```python
from build123d import *

# Parameters (mm, degrees)
BOSS_EXTRUDE1_DEPTH = 50.8
DRAFT1_ANGLE        = 2.86
CUT_EXTRUDE1_DEPTH  = 10.16
SKETCH3_W           = 20.078449586
SKETCH3_H           = 5.08
BOSS_EXTRUDE2_DEPTH = 12.7
CUT_EXTRUDE2_START  = -28.101341283
SKETCH4_R           = 1.905
SKETCH4_W           = 5.08
SKETCH4_H           = 14.732
CUT_EXTRUDE2_DEPTH  = 34.466005054
SKETCH5_W           = 15.24
SKETCH5_H           = 14.732
CUT_EXTRUDE3_DEPTH  = 6.35


with BuildPart() as part:
    # Sketch1 → Boss-Extrude1 (new body)
    with BuildSketch(Plane(origin=(0, 0, 0), x_dir=(1, 0, 0), z_dir=(0, 1, 0))):
        Polygon((-20.199224793, 2.212174897), (0, 0), (20.199224793, 2.212174897), (20.199224793, 22.532174897), (-20.199224793, 22.532174897), align=None)
    extrude(amount=-BOSS_EXTRUDE1_DEPTH)

    # Draft1
    draft1_faces = [part.faces().sort_by_distance(p)[0] for p in [
        (10.099612396, -25.4, -1.106087448),
        (-10.099612396, -25.4, -1.106087448),
    ]]
    draft(draft1_faces, Plane(origin=(0, -50.8, 0), x_dir=(0, 0, -1), z_dir=(0, -1, 0)), DRAFT1_ANGLE)

    # Sketch2 → Cut-Extrude1 (cut)
    with BuildSketch(Plane.ZY.offset(20.199224793)):
        Polygon((-22.532174897, -30.48), (-2.212174897, -50.8), (-22.532174897, -50.8), align=None)
    cut_extrude1 = extrude(amount=-CUT_EXTRUDE1_DEPTH, mode=Mode.SUBTRACT)

    # Mirror1: Cut-Extrude1 across plane
    add(cut_extrude1.mirror(Plane.ZY), mode=Mode.SUBTRACT)

    # Sketch3 → Boss-Extrude2 (add)
    with BuildSketch(Plane.XZ.offset(50.8)):
        with Locations((0, -19.992174897)):
            Rectangle(SKETCH3_W, SKETCH3_H)
    extrude(amount=BOSS_EXTRUDE2_DEPTH)

    # Sketch4 → Cut-Extrude2 (cut)
    with BuildSketch(Plane(origin=(-0.275601276, -0.126470659, 2.516497283), x_dir=(0.99407118, -0.005457579, 0.108594221), z_dir=(-0.108731274, -0.04989569, 0.992818176)).offset(CUT_EXTRUDE2_START)):
        with Locations((-9.882603301, -15.834429405)):
            Circle(SKETCH4_R)
        with Locations((-9.882603301, -34.884429405)):
            Circle(SKETCH4_R)
        with Locations((-4.802603301, -25.359429405)):
            Rectangle(SKETCH4_W, SKETCH4_H)
    cut_extrude2 = extrude(amount=CUT_EXTRUDE2_DEPTH, mode=Mode.SUBTRACT)

    # Sketch5 → Cut-Extrude3 (cut)
    with BuildSketch(Plane(origin=(-0.275601276, -0.126470659, 2.516497283), x_dir=(0.99407118, -0.005457579, 0.108594221), z_dir=(-0.108731274, -0.04989569, 0.992818176))):
        with Locations((-9.882603301, -25.359429405)):
            Rectangle(SKETCH5_W, SKETCH5_H)
    cut_extrude3 = extrude(amount=-CUT_EXTRUDE3_DEPTH, mode=Mode.SUBTRACT)

    # Mirror2: Cut-Extrude2, Cut-Extrude3 across plane
    add(cut_extrude2.mirror(Plane.ZY), mode=Mode.SUBTRACT)
    add(cut_extrude3.mirror(Plane.ZY), mode=Mode.SUBTRACT)


solid = part.part
```
The model under review builds one solid part; all positions refer to its coordinate system, in mm. A direction names the side the tool comes from. Coordinates: 2 decimals unless noted, no trailing zeros. Write each loop counter-clockwise with the first axis right and the second up, starting at its lowest first coordinate (ties: lowest second). Pieces come first, ordered by that corner, then holes.
1) The part is to be moulded in two halves that separate along X. For faces 1 (the face through (9.263, -36.196, -11.837)), 2 (the face through (-20.199, -19, -11)), 3 (the face through (-10.3, -16.44, -11.45)), 4 (the face through (19.058, -25.044, -0.793)), say which applies: pulls with the +X half, pulls with the -X half, needs draft (parallel to the pull), parting line crosses it, or undercut.
2) To check wall thickness, follow probe 1 along X at (y, z) = (-34, -2.75); probe 2 along X at (y, z) = (-25, -4); probe 3 along Y at (x, z) = (-11, -2). State the ranges of each line that lie inside material, in increasing order.
3) We need section B-B on y = -41.5. State the section outline as (x, z) points, then the cut area to 3 significant figures.
4) We need section A-A on x = -13. State the section outline as (y, z) points, then the cut area to 3 significant figures.
5) Machinability: for faces 5 (the face through (15.19, -40.5, -12.51)), 6 (the face through (-1.14, -25.04, 1.17)), 7 (the face through (-10.039, -47, -17)), which of the approach directions +Z, -Z, +X, -X, +Y, -Y give a long, thin tool a straight path to every point of the face, cutting with its end or side? Answer none if there is none.
6) We need section C-C on z = -9. Count the separate pieces of the cut face and the enclosed holes in it, then the cut area to 3 significant figures.
7) Clearance check with flat-ended pins moving along their axes: pin 1 Ø5 at (x, z) = (8.5, -11.5) entering from -Y; pin 2 Ø4 at (x, y) = (5, -60) entering from +Z; pin 3 Ø6 at (y, z) = (-51, -17) entering from -X. State where each tip first meets the part, or that it passes through.
Answer list:
1. face 1: undercut
1. face 2: pulls with the -X half
1. face 3: undercut
1. face 4: pulls with the +X half
2. probe 1: x = -20.2 to -11.57, -8.08 to 8.08, 11.57 to 20.2
2. probe 2: x = -20.2 to -17.31, -1.98 to 1.98, 17.31 to 20.2
2. probe 3: y = -50.8 to -36.41, -33.26 to -32.67, -17.92 to -17.26, -14.27 to 0
3. outline: (-20.2, -11.51) - (-10.04, -11.51) - (-10.04, -22.53) - (10.04, -22.53) - (10.04, -11.51) - (20.2, -11.51) - (20.2, -1.74) - (0, 0.47) - (-20.2, -1.74) - close
3. area: 661 mm2
4. outline: (-50.8, -2.21) - (-30.48, -22.53) - (0, -22.53) - (0, 1.13) - (-18.03, 0.22) - (-17.71, -6.16) - (-32.42, -6.9) - (-32.74, -0.52) - (-50.8, -1.42) - close
4. area: 837 mm2
5. face 5: -Z, +X, -Y
5. face 6: +Z, -X, -Y
5. face 7: -Z, -X, -Y
6. separate pieces: 1
6. enclosed holes: 6
6. area: 1,720 mm2
7. pin 1: stops at y = -50.8
7. pin 2: stops at z = -17.45
7. pin 3: stops at x = -10.04
